```python
from build123d import *

# Parameters (mm, degrees)
SKETCH1_W           = 50
SKETCH1_H           = 36
SKETCH1_R           = 1.7
SKETCH1_W_2         = 9
SKETCH1_H_2         = 9
BOSS_EXTRUDE1_DEPTH = 3.175


with BuildPart() as part:
    # Sketch1 → Boss-Extrude1 (new body)
    with BuildSketch(Plane(origin=(0, 0, 0), x_dir=(1, 0, 0), z_dir=(0, 1, 0))):
        with Locations((25, 18)):
            Rectangle(SKETCH1_W, SKETCH1_H)
        with Locations((5, 5)):
            Circle(SKETCH1_R, mode=Mode.SUBTRACT)
        with Locations((5, 31)):
            Circle(SKETCH1_R, mode=Mode.SUBTRACT)
        with Locations((45, 31)):
            Circle(SKETCH1_R, mode=Mode.SUBTRACT)
        with Locations((45, 5)):
            Circle(SKETCH1_R, mode=Mode.SUBTRACT)
        with Locations((15, 7.3)):
            Rectangle(SKETCH1_W_2, SKETCH1_H_2, mode=Mode.SUBTRACT)
        with Locations((25, 7.3)):
            Rectangle(SKETCH1_W_2, SKETCH1_H_2, mode=Mode.SUBTRACT)
        with Locations((35, 7.3)):
            Rectangle(SKETCH1_W_2, SKETCH1_H_2, mode=Mode.SUBTRACT)
        with Locations((25, 17.3)):
            Rectangle(SKETCH1_W_2, SKETCH1_H_2, mode=Mode.SUBTRACT)
        with Locations((35, 17.3)):
            Rectangle(SKETCH1_W_2, SKETCH1_H_2, mode=Mode.SUBTRACT)
        with Locations((25, 27.3)):
            Rectangle(SKETCH1_W_2, SKETCH1_H_2, mode=Mode.SUBTRACT)
        with Locations((35, 27.3)):
            Rectangle(SKETCH1_W_2, SKETCH1_H_2, mode=Mode.SUBTRACT)
        with Locations((15, 17.3)):
            Rectangle(SKETCH1_W_2, SKETCH1_H_2, mode=Mode.SUBTRACT)
        with Locations((15, 27.3)):
            Rectangle(SKETCH1_W_2, SKETCH1_H_2, mode=Mode.SUBTRACT)
    extrude(amount=BOSS_EXTRUDE1_DEPTH)


solid = part.part
```
Read the model definition and answer for the solid it produces. Units are mm, in the model's axes. A direction names the side the tool comes from. Round coordinates to 2 decimals unless told otherwise and drop trailing zeros. Write each loop counter-clockwise with the first axis right and the second up, starting at its lowest first coordinate (ties: lowest second). Pieces come first, ordered by that corner, then holes. Notation, with made-up numbers: M 23,-3 L 82,-3 A11 cw 82,16 Z; hole C 85.5,-29 d3. An arc over 180 degrees is marked long. One line per item, written item: value.
Q1. Find section A-A on x = 38.5. Write down the section's boundary in (y, z) (3 decimals).
Data:
outline: M 0,-36 L 3.175,-36 L 3.175,-31.8 L 0,-31.8 Z; M 0,-22.8 L 3.175,-22.8 L 3.175,-21.8 L 0,-21.8 Z; M 0,-12.8 L 3.175,-12.8 L 3.175,-11.8 L 0,-11.8 Z; M 0,-2.8 L 3.175,-2.8 L 3.175,0 L 0,0 Z
Q2. For a pull along X with two mould halves and no side action, classify faces 1 (the flat face through (25, 2, -2.8)), 2 (the flat face through (25, 2, -11.8)), 3 (the flat face through (25, 0, -22)), 4 (the flat face through (0, 2, -18)) as +X half, -X half, draft (parallel to the pull), parting line (faces both ways), or undercut.
Data:
face 1: undercut
face 2: undercut
face 3: draft
face 4: -X half
Q3. Find section B-B on z = -15.5. Write down the section's boundary in (x, y) (3 decimals).
Data:
outline: M 0,0 L 10.5,0 L 10.5,3.175 L 0,3.175 Z; M 19.5,0 L 20.5,0 L 20.5,3.175 L 19.5,3.175 Z; M 29.5,0 L 30.5,0 L 30.5,3.175 L 29.5,3.175 Z; M 39.5,0 L 50,0 L 50,3.175 L 39.5,3.175 Z
Q4. Find section D-D on x = 5. Write down the section's boundary in (y, z) (3 decimals).
Data:
outline: M 0,-36 L 3.175,-36 L 3.175,-32.7 L 0,-32.7 Z; M 0,-29.3 L 3.175,-29.3 L 3.175,-6.7 L 0,-6.7 Z; M 0,-3.3 L 3.175,-3.3 L 3.175,0 L 0,0 Z
Q5. Which of the six approach directions +Z, -Z, +X, -X, +Y, -Y give full straight-line access (tool end or side, diameter ignored) to faces 5 (the flat face through (29.5, 2, -27)), 6 (the flat face through (25, 2, 0))?
Data:
face 5: +Y, -Y
face 6: +Z, +X, -X, +Y, -Y
Q6. A flat-ended cylindrical pin translates along its axis: pin 1 Ø3 at (x, z) = (34.5, -15.5) entering from -Y. Find the tip coordinate at first contact, or state that the pin passes through.
Data:
pin 1: through
Q7. Straight lines are drawn through the part: line 1 (Z direction, x = 27, y = 1.2); line 2 (Z direction, x = 5, y = 2.45); line 3 (X direction, y = 0.9, z = -5). For each, find the intervals that lie inside material, in ascending order. Write a range as [from, to].
Data:
line 1: [-36, -31.8], [-22.8, -21.8], [-12.8, -11.8], [-2.8, 0]
line 2: [-36, -32.7], [-29.3, -6.7], [-3.3, 0]
line 3: [0, 3.3], [6.7, 10.5], [19.5, 20.5], [29.5, 30.5], [39.5, 43.3], [46.7, 50]
Q8. Find section C-C on z = -31. Write down the section's boundary in (x, y) (3 decimals).
Data:
outline: M 0,0 L 3.3,0 L 3.3,3.175 L 0,3.175 Z; M 6.7,0 L 10.5,0 L 10.5,3.175 L 6.7,3.175 Z; M 19.5,0 L 20.5,0 L 20.5,3.175 L 19.5,3.175 Z; M 29.5,0 L 30.5,0 L 30.5,3.175 L 29.5,3.175 Z; M 39.5,0 L 43.3,0 L 43.3,3.175 L 39.5,3.175 Z; M 46.7,0 L 50,0 L 50,3.175 L 46.7,3.175 Z
